Can you work these out from the model? Positions are in its coordinate system, mm. Round coordinates to 2 decimals unless told otherwise and drop trailing zeros. Write each loop counter-clockwise with the first axis right and the second up, starting at its lowest first coordinate (ties: lowest second). Pieces come first, ordered by that corner, then holes. Notation, with made-up numbers: M 41,64.5 L 82,64.5 A24 cw 82,101.5 Z; hole C -39,-0.75 d3. An arc over 180 degrees is marked long. Answer in a Markdown table with one row per item. Add a question column.
(1) Suppose I cut it at A-A, the plane y = -11.5. Write out the boundary of the cut face in (x, z).
(2) Suppose I cut it at C-C, the plane z = 0.65. Count the separate pieces of the cut face and the enclosed holes in it, then the cut area to 3 significant figures.
(3) If I drill on probe 1 along Y at (x, z) = (36, 0.55); probe 2 along X at (y, z) = (-19, 0.7); probe 3 along Y at (x, z) = (29, 0.75), over which ranges is the centre line in solid material (lowest first)?
(4) Suppose I cut it at B-B, the plane x = 21. Write out the boundary of the cut face in (y, z), then the cut area to 3 significant figures.
from build123d import *

# Parameters (mm, degrees)
EXTRUDE_1_DEPTH     = 1
CUT_EXTRUDE_4_DEPTH = 54.935146241
SKETCH_4_R          = 1.5
CUT_EXTRUDE_5_DEPTH = 54.935146241
CUT_EXTRUDE1_START  = -1
CUT_EXTRUDE1_DEPTH  = 1


with BuildPart() as part:
    # Эскиз1 → Бобышка-Вытянуть1 (new body)
    with BuildSketch(Plane.XY):
        Polygon((-49, 5.839183832), (-49, -22.516660498), (49, -22.516660498), (49, 5.839183832), (49, 15.839183832), (-49, 15.839183832), align=None)
    extrude(amount=EXTRUDE_1_DEPTH)

    # Эскиз2 → Вырез-Вытянуть4 (cut, through all)
    with BuildSketch(Plane(origin=(0, 0, 0), x_dir=(-1, 0, 0), z_dir=(0, 0, -1))):
        with BuildLine():
            Line((27.226146034, -9.122134253), (15.739905482, -9.122134253))
            ThreePointArc((15.739905482, -9.122134253), (15.10500819, -9.461530461), (14.917793913, -10.156681647))
            Line((14.917793913, -10.156681647), (17.442090319, -18.930924047))
            ThreePointArc((17.442090319, -18.930924047), (18.050493328, -19.909298147), (19.122649731, -20.331021695))
            Line((19.122649731, -20.331021695), (30.826843589, -20.331021695))
            ThreePointArc((30.826843589, -20.331021695), (31.459345435, -19.990005133), (31.64325008, -19.295361367))
            Line((31.64325008, -19.295361367), (29.100959308, -10.488607797))
            ThreePointArc((29.100959308, -10.488607797), (28.40806584, -9.469896887), (27.226146034, -9.122134253))
        make_face()
        with BuildLine():
            Line((-31.64325008, -19.295361367), (-29.100959308, -10.488607797))
            ThreePointArc((-29.100959308, -10.488607797), (-28.40806584, -9.469896887), (-27.226146034, -9.122134253))
            Line((-27.226146034, -9.122134253), (-15.739905482, -9.122134253))
            ThreePointArc((-15.739905482, -9.122134253), (-15.10500819, -9.461530461), (-14.917793913, -10.156681647))
            Line((-14.917793913, -10.156681647), (-17.442090319, -18.930924047))
            ThreePointArc((-17.442090319, -18.930924047), (-18.050493328, -19.909298147), (-19.122649731, -20.331021695))
            Line((-19.122649731, -20.331021695), (-30.826843589, -20.331021695))
            ThreePointArc((-30.826843589, -20.331021695), (-31.459345435, -19.990005133), (-31.64325008, -19.295361367))
        make_face()
    extrude(amount=-CUT_EXTRUDE_4_DEPTH, mode=Mode.SUBTRACT)

    # Эскиз4 → Вырез-Вытянуть5 (cut, through all)
    with BuildSketch(Plane(origin=(0, 0, 0), x_dir=(-1, 0, 0), z_dir=(0, 0, -1))):
        with Locations((36, -7.524952718)):
            Circle(SKETCH_4_R)
        with Locations((-36, -7.524952718)):
            Circle(SKETCH_4_R)
    extrude(amount=-CUT_EXTRUDE_5_DEPTH, mode=Mode.SUBTRACT)

    # Sketch3 → Cut-Extrude1 (cut)
    with BuildSketch(Plane.XY.offset(1).offset(CUT_EXTRUDE1_START)):
        with BuildLine():
            Line((8.652344227, -7.068131311), (12.085677561, -18.961546856))
            add(Edge.make_bspline(
                [(12.085677561, -18.961546856), (12.485677561, -20.347187502), (13.871318207, -20.347187502)],
                knots=[0.857071948, 0.857071948, 0.857071948, 2.427868275, 2.427868275, 2.427868275], degree=2, weights=[1, 0.707106781, 1]))
            Line((13.871318207, -20.347187502), (32.461996875, -20.347187502))
            add(Edge.make_bspline(
                [(32.461996875, -20.347187502), (33.393769403, -20.347187502), (33.496157418, -19.484255682)],
                knots=[2.427868275, 2.427868275, 2.427868275, 3.611858299, 3.611858299, 3.611858299], degree=2, weights=[1, 0.829829079, 1]))
            add(Edge.make_bspline(
                [(33.496157418, -19.484255682), (33.529743577, -19.201189685), (33.607326061, -18.923570429), (33.853252735, -18.417152493), (34.025349409, -18.183932413), (34.436238564, -17.8036127), (34.681879478, -17.649935655), (35.200024528, -17.435065661), (35.479061866, -17.369439067), (35.76148791, -17.34207634)],
                knots=[0, 0, 0, 0, 0.25, 0.25, 0.5, 0.5, 0.75, 0.75, 1, 1, 1, 1], degree=3))
            add(Edge.make_bspline(
                [(35.76148791, -17.34207634), (36.181169226, -17.301415694), (36.592378309, -17.212108423), (37.170380488, -16.959028015), (37.354968395, -16.854344533), (37.687544868, -16.599797528), (37.83830967, -16.446579579), (38.076557482, -16.101495837), (38.166209489, -15.905573827), (38.271501218, -15.499696694), (38.288800836, -15.285469364), (38.263278752, -14.867475934), (38.220734772, -14.657932914), (38.094284502, -14.258193956), (38.010543981, -14.065974434), (37.910619322, -13.879789794)],
                knots=[0, 0, 0, 0, 0.25, 0.25, 0.375, 0.375, 0.5, 0.5, 0.625, 0.625, 0.75, 0.75, 0.875, 0.875, 1, 1, 1, 1], degree=3))
            Line((37.910619322, -13.879789794), (35.170885606, -8.774980446))
            ThreePointArc((35.170885606, -8.774980446), (34.803783463, -8.429975368), (34.571610551, -7.982886756))
            ThreePointArc((34.571610551, -7.982886756), (34.527886571, -7.812845152), (34.504331156, -7.638859302))
            add(Edge.make_bspline(
                [(34.504331156, -7.638859302), (33.03670289, -5.782259548), (30.630891119, -5.783194379)],
                knots=[4.00651056, 4.00651056, 4.00651056, 5.38030343, 5.38030343, 5.38030343], degree=2, weights=[1, 0.773217832, 1]))
            Line((30.630891119, -5.783194379), (28.778313515, -5.783914238))
            add(Edge.make_bspline(
                [(28.778313515, -5.783914238), (28.498733332, -5.682490665), (28.228663541, -5.682490665)],
                knots=[5.18447533, 5.18447533, 5.18447533, 5.569460928, 5.569460928, 5.569460928], degree=2, weights=[1, 0.981530397, 1]))
            Line((28.228663541, -5.682490665), (9.637984874, -5.682490665))
            add(Edge.make_bspline(
                [(9.637984874, -5.682490665), (8.252344227, -5.682490665), (8.652344227, -7.068131311)],
                knots=[5.569460928, 5.569460928, 5.569460928, 7.140257255, 7.140257255, 7.140257255], degree=2, weights=[1, 0.707106781, 1]))
        make_face()
        with BuildLine():
            Line((-35.170885606, -8.774980446), (-37.925052204, -13.906681863))
            add(Edge.make_bspline(
                [(-37.925052204, -13.906681863), (-38.025225081, -14.093328995), (-38.109806595, -14.28778394), (-38.235924368, -14.687324932), (-38.278394681, -14.895918794), (-38.297414091, -15.212202185), (-38.296322734, -15.317469634), (-38.277441195, -15.527644209), (-38.259343447, -15.633280004), (-38.205994928, -15.836909506), (-38.170798519, -15.935630825), (-38.082894213, -16.126717018), (-38.029532599, -16.219817403), (-37.849055501, -16.479499021), (-37.698892817, -16.631115336), (-37.362837335, -16.886481906), (-37.179664999, -16.989484869), (-36.595923377, -17.242719775), (-36.186794345, -17.329699001), (-35.766265682, -17.369273893)],
                knots=[0, 0, 0, 0, 0.125, 0.125, 0.25, 0.25, 0.3125, 0.3125, 0.375, 0.375, 0.4375, 0.4375, 0.5, 0.5, 0.625, 0.625, 0.75, 0.75, 1, 1, 1, 1], degree=3))
            add(Edge.make_bspline(
                [(-33.495182661, -19.492227082), (-33.738478544, -17.560103824), (-35.766265682, -17.369273893)],
                knots=[5.81913938, 5.81913938, 5.81913938, 6.905546226, 6.905546226, 6.905546226], degree=2, weights=[1, 0.856057288, 1]))
            add(Edge.make_bspline(
                [(-33.495182661, -19.492227082), (-33.387524752, -20.347187502), (-32.461996875, -20.347187502)],
                knots=[2.677546726, 2.677546726, 2.677546726, 3.855317033, 3.855317033, 3.855317033], degree=2, weights=[1, 0.83156042, 1]))
            Line((-32.461996875, -20.347187502), (-13.871318207, -20.347187502))
            add(Edge.make_bspline(
                [(-13.871318207, -20.347187502), (-12.46794332, -20.347187502), (-12.080702928, -18.943926093)],
                knots=[3.855317033, 3.855317033, 3.855317033, 5.438830393, 5.438830393, 5.438830393], degree=2, weights=[1, 0.702596367, 1]))
            Line((-12.080702928, -18.943926093), (-8.83075434, -7.166932971))
            add(Edge.make_bspline(
                [(-8.83075434, -7.166932971), (-8.45309236, -5.798381309), (-9.82190813, -5.798913193)],
                knots=[5.438830393, 5.438830393, 5.438830393, 6.997298301, 6.997298301, 6.997298301], degree=2, weights=[1, 0.711452073, 1]))
            Line((-9.82190813, -5.798913193), (-30.645016113, -5.807004464))
            add(Edge.make_bspline(
                [(-30.645016113, -5.807004464), (-33.032902471, -5.807932329), (-34.505069218, -7.648167801)],
                knots=[0.90305787, 0.90305787, 0.90305787, 2.269113721, 2.269113721, 2.269113721], degree=2, weights=[1, 0.775665219, 1]))
            ThreePointArc((-34.505069218, -7.648167801), (-34.53118454, -7.829224215), (-34.579145022, -8.005755309))
            ThreePointArc((-34.579145022, -8.005755309), (-34.811085633, -8.43954696), (-35.170885606, -8.774980446))
        make_face()
    extrude(amount=CUT_EXTRUDE1_DEPTH, mode=Mode.SUBTRACT)


solid = part.part
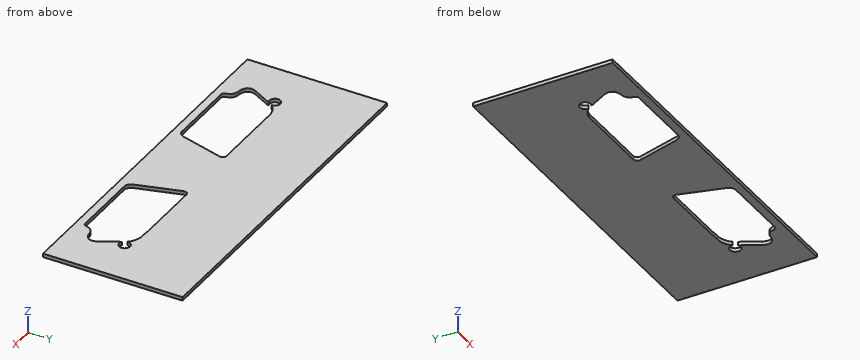
Calculated:
| question | item | result |
|---|---|---|
| 1 | outline | M -49,0 L -36.63,0 L -36.63,1 L -49,1 Z; M -10.03,0 L 9.93,0 L 9.93,1 L -10.03,1 Z; M 36.63,0 L 49,0 L 49,1 L 36.63,1 Z |
| 2 | separate pieces | 1 |
| 2 | enclosed holes | 2 |
| 2 | area | 3,010 mm² |
| 3 | probe 1 | -22.52 to -17.31, -10.32 to -9.02, -6.02 to 15.84 |
| 3 | probe 2 | -49 to -33.6, -12.1 to 12.1, 33.6 to 49 |
| 3 | probe 3 | -22.52 to -20.35, -5.78 to 15.84 |
| 4 | outline | M -22.52,0 L -20.35,0 L -20.35,1 L -22.52,1 Z; M -5.68,0 L 15.84,0 L 15.84,1 L -5.68,1 Z |
| 4 | area | 23.7 mm² |
